Design review of the part built by this model. Coordinates are the model's own, in mm. Face numbers are marked on the shaded views. A direction names the side the tool comes from. Round coordinates to 2 decimals unless told otherwise and drop trailing zeros. Order: outer loops, then holes, each group sorted by start corner. A loop starts at its lowest first (then second) coordinate and runs counter-clockwise, first axis right, second up. Notation, with made-up numbers: M 77.5,24.25 L 109.5,24.25 A24 ccw 109.5,41.25 Z; hole C 47.25,11 d1. An arc over 180 degrees is marked long. Write each question's results on one line, items separated by ' | '. Start each with the question number.
Item 1: Take a section at B-B, the plane x = 12. Write out the cut boundary in (y, z).
Item 2: Wall thickness on line 1 (Z direction, x = -10.5, y = -2); line 2 (X direction, y = 4.25, z = -2.5); line 3 (X direction, y = 1.5, z = -3): over which ranges is each line inside the solid? List them lowest first. Write a range as [from, to].
Item 3: Take a section at A-A, the plane z = 4.5. Write out the cut boundary in (x, y).
Item 4: Machinability: for the marked faces 1, 2 and 3, which of the approach directions +Z, -Z, +X, -X, +Y, -Y give a long, thin tool a straight path to every point of the face, cutting with its end or side? Answer none if there is none.
Item 5: The part is to be moulded in two halves that separate along Z. For the marked faces 4, 5, 6 and 7, say which applies: +Z half, -Z half, draft (parallel to the pull), parting line (faces both ways), or undercut.
Item 6: Take a section at D-D, the plane x = -20.5. Write out the cut boundary in (y, z).
Item 7: Clearance check with flat-ended pins moving along their axes: pin 1 (2 mm diameter, centred on y = -2, z = -7.5, fed in from +X); pin 2 (0.9 mm diameter, centred on x = 3, y = -3, fed in from -Z); pin 3 (3 mm diameter, centred on x = 12.5, y = -2, fed in from +Z). State where each tip first meets the part, or that it passes through.
Item 8: Take a section at C-C, the plane z = -1. Write out the cut boundary in (x, y), plus the area to 3 significant figures.
```python
from build123d import *

# Parameters (mm, degrees)
SKETCH1_R           = 3
BOSS_EXTRUDE1_DEPTH = 5
BOSS_EXTRUDE2_DEPTH = 4


with BuildPart() as part:
    # Sketch1 → Boss-Extrude1 (new body)
    with BuildSketch(Plane(origin=(0, 0, 0), x_dir=(1, 0, 0), z_dir=(0, 1, 0))):
        with BuildLine():
            Line((-26.214135995, 14.392719194), (25.785864005, 14.392719194))
            ThreePointArc((25.785864005, 14.392719194), (26.492970786, 14.099825975), (26.785864005, 13.392719194))
            Line((26.785864005, 13.392719194), (26.785864005, -9.607280806))
            ThreePointArc((26.785864005, -9.607280806), (26.492970786, -10.314387587), (25.785864005, -10.607280806))
            Line((25.785864005, -10.607280806), (2.893081301, -10.607280806))
            ThreePointArc((2.893081301, -10.607280806), (2.18597452, -10.314387587), (1.893081301, -9.607280806))
            Line((1.893081301, -9.607280806), (1.893081301, -1.362307791))
            ThreePointArc((1.893081301, -1.362307791), (1.97370849, -0.968920407), (2.202588568, -0.638968461))
            ThreePointArc((2.202588568, -0.638968461), (-0.258950026, 5.392432282), (-2.565241962, -0.700020811))
            ThreePointArc((-2.565241962, -0.700020811), (-2.322726014, -1.035676875), (-2.236986524, -1.440803669))
            Line((-2.236986524, -1.440803669), (-2.236986524, -9.607280806))
            ThreePointArc((-2.236986524, -9.607280806), (-2.529879743, -10.314387587), (-3.236986524, -10.607280806))
            Line((-3.236986524, -10.607280806), (-26.214135995, -10.607280806))
            ThreePointArc((-26.214135995, -10.607280806), (-26.921242776, -10.314387587), (-27.214135995, -9.607280806))
            Line((-27.214135995, -9.607280806), (-27.214135995, 13.392719194))
            ThreePointArc((-27.214135995, 13.392719194), (-26.921242776, 14.099825975), (-26.214135995, 14.392719194))
        make_face()
        with Locations(Location((-22.214135995, 1.892719194, 0), (0, 0, 270))):
            Circle(SKETCH1_R, mode=Mode.SUBTRACT)
        with Locations(Location((21.785864005, 1.892719194, 0), (0, 0, 270))):
            Circle(SKETCH1_R, mode=Mode.SUBTRACT)
    extrude(amount=BOSS_EXTRUDE1_DEPTH)

    # 3DSketch1 → Boss-Extrude2 (add)
    with BuildSketch(Plane(origin=(4.245395627, 0, -4.892719194), x_dir=(-0.9022274497491443, 0, 0.43126051166221485), z_dir=(0, 1, 0))):
        with BuildLine():
            Line((0, 0), (-0.431260512, -0.90222745))
            ThreePointArc((-0.431260512, -0.90222745), (-0.451605977, -1.284369663), (-0.195777043, -1.56897143))
            Line((-0.195777043, -1.56897143), (6.416167911, -4.72945027))
            ThreePointArc((6.416167911, -4.72945027), (6.798310124, -4.749795735), (7.082911891, -4.493966801))
            Line((7.082911891, -4.493966801), (7.514172403, -3.591739351))
            ThreePointArc((7.514172403, -3.591739351), (7.79877417, -3.335910417), (8.180916384, -3.356255882))
            Line((8.180916384, -3.356255882), (19.358269109, -8.698978337))
            ThreePointArc((19.358269109, -8.698978337), (19.482317491, -8.836978321), (19.472452219, -9.022274497))
            Line((19.472452219, -9.022274497), (17.525262711, -13.095932476))
            ThreePointArc((17.525262711, -13.095932476), (17.387262727, -13.219980858), (17.201966551, -13.210115586))
            Line((17.201966551, -13.210115586), (-13.036287471, 1.24362876))
            ThreePointArc((-13.036287471, 1.24362876), (-13.160335853, 1.381628744), (-13.150470581, 1.56692492))
            Line((-13.150470581, 1.56692492), (-11.203281073, 5.640582899))
            ThreePointArc((-11.203281073, 5.640582899), (-11.065281089, 5.764631281), (-10.879984912, 5.754766009))
            Line((-10.879984912, 5.754766009), (-0.235483469, 0.666743981))
            ThreePointArc((-0.235483469, 0.666743981), (0.020345465, 0.382142214), (0, 0))
        make_face()
        with BuildLine():
            Line((-8.723682354, 10.265903258), (2.335421133, 4.979703387))
            ThreePointArc((2.335421133, 4.979703387), (2.717563346, 4.959357922), (3.002165113, 5.215186856))
            Line((3.002165113, 5.215186856), (3.3288691, 5.898674671))
            ThreePointArc((3.3288691, 5.898674671), (3.466869084, 6.022723053), (3.65216526, 6.012857781))
            Line((3.65216526, 6.012857781), (4.690032412, 5.516762124))
            ThreePointArc((4.690032412, 5.516762124), (5.072174626, 5.496416659), (5.356776393, 5.752245593))
            Line((5.356776393, 5.752245593), (6.546001403, 8.240188308))
            ThreePointArc((6.546001403, 8.240188308), (6.555866675, 8.425484484), (6.431818293, 8.563484468))
            Line((6.431818293, 8.563484468), (-6.567379796, 14.777040507))
            ThreePointArc((-6.567379796, 14.777040507), (-6.752675972, 14.786905779), (-6.890675956, 14.662857397))
            Line((-6.890675956, 14.662857397), (-8.837865464, 10.589199418))
            ThreePointArc((-8.837865464, 10.589199418), (-8.847730736, 10.403903241), (-8.723682354, 10.265903258))
        make_face()
        with BuildLine():
            Line((21.837867827, -4.073657979), (23.785057336, 0))
            ThreePointArc((23.785057336, 0), (23.794922608, 0.185296176), (23.670874226, 0.32329616))
            Line((23.670874226, 0.32329616), (10.595558124, 6.573236254))
            ThreePointArc((10.595558124, 6.573236254), (10.410261948, 6.583101526), (10.272261964, 6.459053144))
            Line((10.272261964, 6.459053144), (9.083036954, 3.97111043))
            ThreePointArc((9.083036954, 3.97111043), (9.062691489, 3.588968216), (9.318520423, 3.304366449))
            Line((9.318520423, 3.304366449), (10.432505588, 2.771886738))
            ThreePointArc((10.432505588, 2.771886738), (10.55655397, 2.633886754), (10.546688698, 2.448590577))
            Line((10.546688698, 2.448590577), (10.219984711, 1.765102763))
            ThreePointArc((10.219984711, 1.765102763), (10.199639246, 1.382960549), (10.45546818, 1.098358782))
            Line((10.45546818, 1.098358782), (21.514571667, -4.187841089))
            ThreePointArc((21.514571667, -4.187841089), (21.699867844, -4.197706361), (21.837867827, -4.073657979))
        make_face()
    extrude(amount=-BOSS_EXTRUDE2_DEPTH)


solid = part.part
```
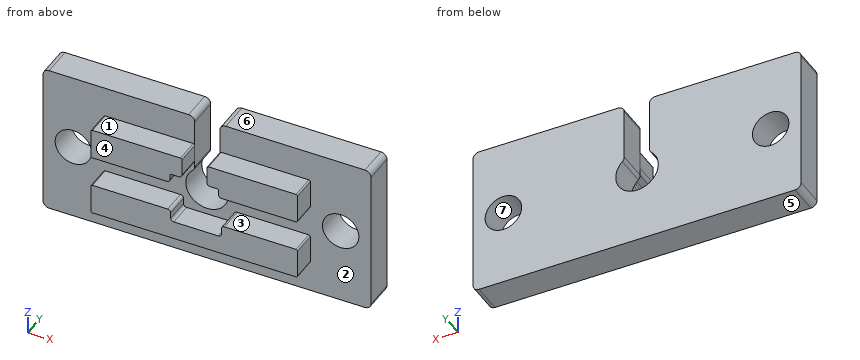
Results list:
1) outline: M -4,-9.39 L 0,-9.39 L 0,-14.39 L 5,-14.39 L 5,10.61 L 0,10.61 L 0,5.61 L -4,5.61 L -4,0.61 L 0,0.61 L 0,-4.39 L -4,-4.39 Z
2) line 1: [-9.39, -4.39], [0.61, 5.61] | line 2: [-27.21, -25.15], [-19.28, -3.66], [3.23, 18.85], [24.72, 26.79] | line 3: [-27.21, -25], [-19.43, -3.53], [3.11, 19], [24.57, 26.79]
3) outline: M -27.21,0 L -17.21,0 L -17.21,-4 L -2.24,-4 L -2.24,5 L -27.21,5 Z; M 1.89,-4 L 16.79,-4 L 16.79,0 L 26.79,0 L 26.79,5 L 1.89,5 Z
4) face 1: +Z, +X, -X, -Y | face 2: -Y | face 3: +X, -X, -Y
5) face 4: draft | face 5: -Z half | face 6: +Z half | face 7: undercut
6) outline: M 0,-14.39 L 5,-14.39 L 5,-4.35 L 0,-4.35 Z; M 0,0.57 L 5,0.57 L 5,10.61 L 0,10.61 Z
7) pin 1: x = 16.79 | pin 2: z = -9.39 | pin 3: z = 5.61
8) outline: M -27.21,0 L -25.08,0 L -25.08,5 L -27.21,5 Z; M -19.35,0 L -3.6,0 L -3.6,5 L -19.35,5 Z; M 3.17,0 L 18.92,0 L 18.92,5 L 3.17,5 Z; M 24.65,0 L 26.79,0 L 26.79,5 L 24.65,5 Z | area: 179 mm²
